Read the model definition and answer for the solid it produces. Units are mm, in the model's axes. Face numbers are marked on the shaded views. A direction names the side the tool comes from. Coordinates: 2 decimals unless noted, no trailing zeros. Loops run counter-clockwise (first coordinate to the right, second up) from the corner with the lowest first, then second, coordinate; pieces in that order, holes last. Notation, with made-up numbers: (46, -29.75) -> (78, -29.75) arc R29 cw to (78, -7.75) -> close; hole circle Ø4 at (34.5, -40). An arc over 180 degrees is marked (long way). Answer as a JSON object with one key per item and string values. Group by question number.
1) Determine the mould class of the marked faces 3 and 4 for opening direction Y: released by +Y, released by -Y, zero draft, split by the parting line, or undercut.
2) Consider probe 1 along Y at (x, z) = (3.55, -2.75); probe 2 along Y at (x, z) = (1.3, 3.75); probe 3 along Y at (x, z) = (1.9, 1.25). Determine where each line is inside the solid, lowest interval first. Write a range as [from, to].
3) Flat-ended cylindrical pins translate along their axes: P1, Ø0.5, axis at x = 2, z = -2.5, coming from the -Y side; P2, Ø1, axis at x = 2, z = 3.5, coming from the +Y side; P3, Ø1.5, axis at x = 2, y = 31, coming from the -Z side. Find the tip coordinate at first contact, or state that the pin passes through.
4) Section A-A, the plane x = 1.85 is taken. Give the vertices of the cut face in (y, z).
5) Which of the six approach directions +Z, -Z, +X, -X, +Y, -Y give full straight-line access (tool end or side, diameter ignored) to the marked faces 1 and 2?
from build123d import *

# Parameters (mm, degrees)
BOSS_EXTRUDE1_DEPTH = 4
FILLET1_R           = 1
FILLET2_R           = 1


with BuildPart() as part:
    # Sketch1 → Boss-Extrude1 (new body)
    with BuildSketch(Plane.YZ):
        Polygon((-33.5, -2), (-33.5, 2), (-29.5, 2), (-29.5, 4), (-2.5, 4), (-2.5, 2), (2.5, 2), (2.5, 4), (29.5, 4), (29.5, 2), (33.5, 2), (33.5, -2), (29.5, -2), (29.5, -4), (2.5, -4), (2.5, -2), (-2.5, -2), (-2.5, -4), (-29.5, -4), (-29.5, -2), align=None)
    extrude(amount=BOSS_EXTRUDE1_DEPTH)

    # Fillet1
    fillet1_edges = [part.edges().sort_by_distance(p)[0] for p in [
        (2, -2.5, 4),
        (2, 2.5, 4),
        (2, 2.5, -4),
        (2, -2.5, -4),
    ]]
    fillet(fillet1_edges, radius=FILLET1_R)

    # Fillet2
    fillet2_edges = [part.edges().sort_by_distance(p)[0] for p in [
        (2, -33.5, -2),
        (2, -33.5, 2),
        (2, 33.5, 2),
        (2, 33.5, -2),
    ]]
    fillet(fillet2_edges, radius=FILLET2_R)


solid = part.part
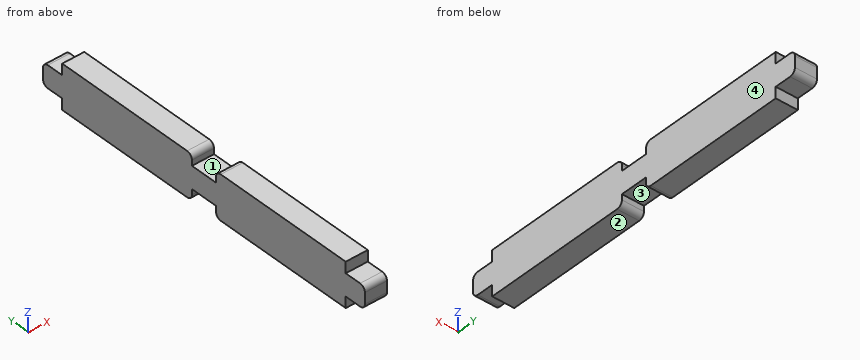
Determined:
{
 "1": {"face 3": "undercut", "face 4": "zero draft"},
 "2": {"probe 1": "[-29.5, -2.5], [2.5, 29.5]", "probe 2": "[-29.5, -2.84], [2.84, 29.5]", "probe 3": "[-33.47, 33.47]"},
 "3": {"P1": "y = -29.5", "P2": "y = 29.5", "P3": "z = -2"},
 "4": {"outline": "(-33.5, -1) arc R1 ccw to (-32.5, -2) -> (-29.5, -2) -> (-29.5, -4) -> (-3.5, -4) arc R1 ccw to (-2.5, -3) -> (-2.5, -2) -> (2.5, -2) -> (2.5, -3) arc R1 ccw to (3.5, -4) -> (29.5, -4) -> (29.5, -2) -> (32.5, -2) arc R1 ccw to (33.5, -1) -> (33.5, 1) arc R1 ccw to (32.5, 2) -> (29.5, 2) -> (29.5, 4) -> (3.5, 4) arc R1 ccw to (2.5, 3) -> (2.5, 2) -> (-2.5, 2) -> (-2.5, 3) arc R1 ccw to (-3.5, 4) -> (-29.5, 4) -> (-29.5, 2) -> (-32.5, 2) arc R1 ccw to (-33.5, 1) -> close"},
 "5": {"face 1": "+Z, +X, -X", "face 2": "-Z, +X, -X, +Y, -Y"}
}
